Geometry check sheet. Reference: drawing and pictorial views, mm from the part's lowest x, y, z. Coordinates: 2 decimals unless noted, no trailing zeros. Loops run counter-clockwise (first coordinate to the right, second up) from the corner with the lowest first, then second, coordinate; pieces in that order, holes last.
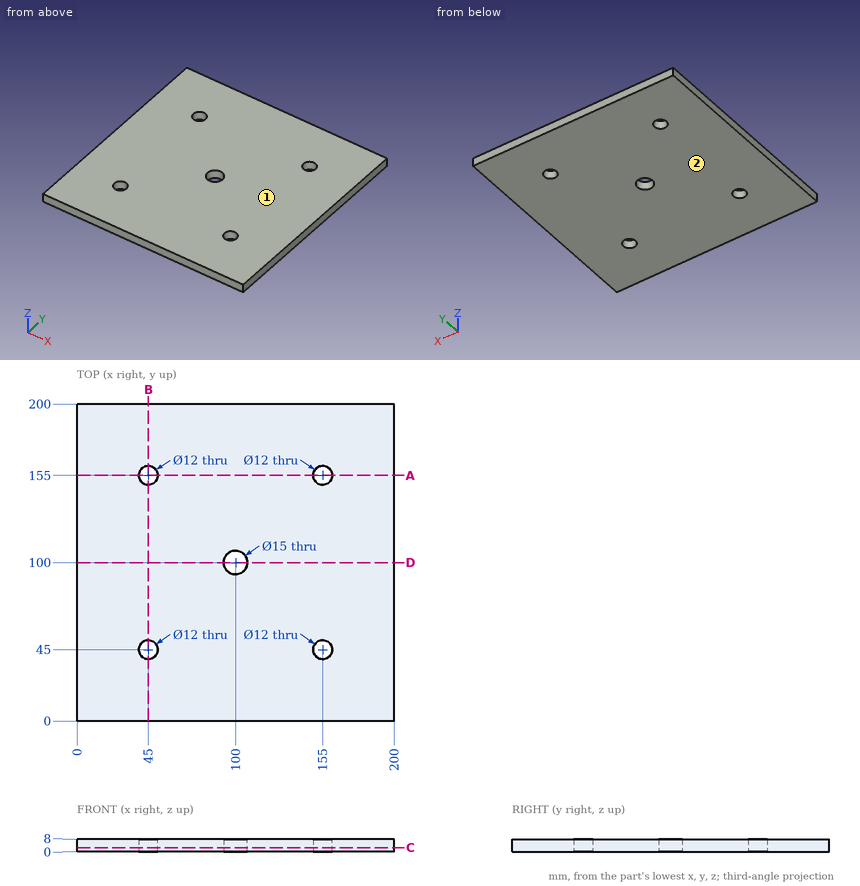
1) Mould release check, pull along Z, two halves, no side actions. Record for the marked faces 1 and 2: +Z half, -Z half, draft (parallel to the pull), parting line (faces both ways), or undercut.
Data:
face 1: +Z half
face 2: -Z half
2) Material ranges on probe 1 along Y at (x, z) = (45, 5.25); probe 2 along X at (y, z) = (100, 6.5), recorded low to high.
Data:
probe 1: y = 0 to 39, 51 to 149, 161 to 200
probe 2: x = 0 to 92.5, 107.5 to 200
3) Section check C-C on z = 2.5. Record the cut outline in (x, y).
Data:
outline: (0, 0) - (200, 0) - (200, 200) - (0, 200) - close; hole circle Ø12 at (45, 45); hole circle Ø12 at (45, 155); hole circle Ø15 at (100, 100); hole circle Ø12 at (155, 45); hole circle Ø12 at (155, 155)
4) Section check A-A on y = 155. Record the cut outline in (x, z).
Data:
outline: (0, 0) - (39, 0) - (39, 8) - (0, 8) - close; (51, 0) - (149, 0) - (149, 8) - (51, 8) - close; (161, 0) - (200, 0) - (200, 8) - (161, 8) - close
5) Section check D-D on y = 100. Record the cut outline in (x, z).
Data:
outline: (0, 0) - (92.5, 0) - (92.5, 8) - (0, 8) - close; (107.5, 0) - (200, 0) - (200, 8) - (107.5, 8) - close
6) Depth check by flat-ended pin: pin 1 (12 mm diameter, centred on x = 36.5, y = 82, fed in from -Z); pin 2 (9.5 mm diameter, centred on x = 155, y = 45, fed in from -Z). Enter the tip coordinate at first touch or a pass-through.
Data:
pin 1: stops at z = 0
pin 2: passes through
